Autodesk Inventor part; units mm, degrees
ref_plane "YZ Plane" through (0, 0, 0) normal (1, 0, 0) x (0, 1, 0)
ref_plane "XZ Plane" through (0, 0, 0) normal (0, 1, 0) x (-1, 0, 0)
ref_plane "XY Plane" through (0, 0, 0) normal (0, 0, 1) x (1, 0, 0)
sketch "Sketch1" plane through (0, 0, 0) normal (0, 1, 0) x (-1, 0, 0)
  line L0 (0, -22.2029) -> (0, 22.4648)
  line L1 (10.56, 0) -> (-1.76, 0)
  line L2 (0, 16.0837) -> (0, -15.8218)
  line L3 (0, -11.9411) -> (8.8, -11.9411)
  line L4 (8.8, -11.9411) -> (8.8, 11.0589)
  line L5 (8.8, 11.0589) -> (3.075, 11.0589)
  line L6 (3.075, 11.0589) -> (3.075, 12.2589)
  line L7 (3.075, 12.2589) -> (1.825, 12.2589)
  line L8 (1.825, 12.2589) -> (1.825, 15.2589)
  line L9 (1.825, 15.2589) -> (0, 15.2589)
  line L10 (0, -11.9411) -> (0, 15.2589)
  line L11 (0, -12.9411) -> (2.35, -12.9411)
  line L12 (2.35, -12.9411) -> (2.35, -11.9411)
  line L13 (0, -11.9411) -> (0, -12.9411)
  point P0 (0, 0)
  dimension "d0" = 17.6
  dimension "d1" = 23
  dimension "d2" = 1
  dimension "d3" = 4.7
  dimension "d4" = 6.15
  dimension "d5" = 3.65
  dimension "d6" = 1.2
  dimension "d7" = 3
revolve "Revolution1" add sketch "Sketch1" angle 360 about axis through (0, 0, -10) along (0, 0, 1)
sketch "Sketch2" plane through (0, 0, 11.0589) normal (0, 0, 1) x (1, 0, 0)
  line L0 (-12.32, 0) -> (12.32, 0)
  circle A0 centre (-5.075, 0) radius 0.725
  circle A1 centre (5.075, 0) radius 0.725
  line L1 (0, -12.32) -> (0, 12.32)
  dimension "d9" = 1.45
  dimension "d10" = 10.15
extrude "Extrusion1" cut sketch "Sketch2" against normal blind 10
sketch "Sketch3" plane through (0, 0, -11.9411) normal (0, 0, -1) x (-1, 0, 0)
  line L0 (12.32, 0) -> (-12.32, 0)
  line L1 (0, -12.32) -> (0, 12.32)
  line L2 (-2, 7) -> (2, 7)
  line L3 (2, 7) -> (2, 5)
  line L4 (2, 5) -> (-2, 5)
  line L5 (-2, 5) -> (-2, 7)
  line L6 (-2, 7) -> (2, 5) construction
  line L7 (2, 7) -> (-2, 5) construction
  line L8 (-2, -7) -> (2, -7)
  line L9 (2, -7) -> (2, -5)
  line L10 (2, -5) -> (-2, -5)
  line L11 (-2, -5) -> (-2, -7)
  line L12 (-2, -7) -> (2, -5) construction
  line L13 (2, -7) -> (-2, -5) construction
  point P0 (0, 6)
  point P1 (0, -6)
  dimension "d13" = 4
  dimension "d14" = 14
  dimension "d15" = 2
extrude "Extrusion2" add sketch "Sketch3" along normal blind 1
sketch "Sketch4" plane through (0, 0, 15.2589) normal (0, 0, 1) x (1, 0, 0)
  circle A0 centre (0, 0) radius 1.825
  line L0 (0, -12.32) -> (0, 12.32)
  line L1 (-12.32, 0) -> (12.32, 0)
  line L2 (-0.4802, 1.7607) -> (0, 0.7709)
  line L3 (0.4802, 1.7607) -> (0, 0.7709)
  line L4 (0, 0) -> (-0.564, 1.7357) construction
  line L5 (0, 0) -> (0.564, 1.7357) construction
  arc A1 (-0.09, 0.9564) -> (0.09, 0.9564) centre (0, 1) ccw
  arc A2 (-0.4431, 1.6842) -> (-0.564, 1.7357) centre (-0.5331, 1.6406) ccw
  arc A3 (0.564, 1.7357) -> (0.4431, 1.6842) centre (0.5331, 1.6406) ccw
  line L6 (0, 1) -> (0, 1.825)
  dimension "d18" = 0.1
  dimension "d19" = 36
  dimension "d22" = 0.1
  dimension "d29" = 0.825
extrude "Extrusion3" cut sketch "Sketch4" against normal up to surface (3 mm away) contours A3 L3 A0 | L3 A1 L0 A0 | L0 A1 L2 A0 | A0 L2 A2
pattern_circular "Circular Pattern1" count 10 over 360 about axis through (0, 0, -10) along (0, 0, 1) of "Extrusion3"
fillet "Fillet1" radius 0.5 1 edges at (8.8, 0, 11.0589)
properties part number "empty"
The model under review builds one solid part; all positions refer to its coordinate system, in mm. A direction names the side the tool comes from. Round coordinates to 2 decimals unless told otherwise and drop trailing zeros. Loops run counter-clockwise (first coordinate to the right, second up) from the corner with the lowest first, then second, coordinate; pieces in that order, holes last. Notation, with made-up numbers: (-31, 18) - (11, 18) arc R20 ccw to (11, 26) - close; hole circle Ø10 at (86.25, -4.75). An arc over 180 degrees is marked (long way). Use a Markdown table: item, result. Add a question column.
Q1. Insertion check: pin 1 Ø1.2 at (x, y) = (-5, 0) entering from +Z; pin 2 Ø9 at (x, y) = (-3.5, 3.5) entering from -Z; pin 3 Ø0.8 at (x, z) = (-0.5, -12.5) entering from -Y; pin 4 Ø1.2 at (x, y) = (5.075, 0) entering from -Z. Each pin has a flat end and moves straight along its axis. Give the tip position at first contact, or say it passes through.
Q2. The part is to be moulded in two halves that separate along X. For faces 1 (the face through (-2, 6, -12.4)), 2 (the face through (0, 6, -12.941)), 3 (the face through (-5, 0, 1.059)), say which applies: pulls with the +X half, pulls with the -X half, needs draft (parallel to the pull), parting line crosses it, or undercut.
Q3. Add section A-A (z = 2). State the section outline as (x, y) points (3 decimals).
Q4. For probe 1 along X at (y, z) = (0, 4.75); probe 2 along Z at (x, y) = (-1.25, -8); probe 3 along Y at (x, z) = (-5.25, 9.5), list the stretches that pass through material, from the lowest coordinate up.
Q5. Machinability: for faces 4 (the face through (4.35, 0.03, 6.13)), 5 (the face through (0, -5, -12.4)), 6 (the face through (0, 7, -12.4)), which of the approach directions +Z, -Z, +X, -X, +Y, -Y give a long, thin tool a straight path to every point of the face, cutting with its end or side? Answer none if there is none.
Worked answers:
| question | item | result |
|---|---|---|
| 1 | pin 1 | z = 1.06 |
| 1 | pin 2 | z = -12.94 |
| 1 | pin 3 | y = -7 |
| 1 | pin 4 | z = -11.94 |
| 2 | face 1 | pulls with the -X half |
| 2 | face 2 | needs draft |
| 2 | face 3 | undercut |
| 3 | outline | circle Ø17.6 at (0, 0); hole circle Ø1.45 at (-5.075, 0); hole circle Ø1.45 at (5.075, 0) |
| 4 | probe 1 | -8.8 to -5.8, -4.35 to 4.35, 5.8 to 8.8 |
| 4 | probe 2 | -11.94 to 11.06 |
| 4 | probe 3 | -7.06 to -0.7, 0.7 to 7.06 |
| 5 | face 4 | +Z |
| 5 | face 5 | -Z, +X, -X |
| 5 | face 6 | -Z, +X, -X, +Y |
